Source: CAD feature listing. Evaluate the final solid. Frame: model axes, mm. Round coordinates to 2 decimals unless told otherwise and drop trailing zeros. Write each loop counter-clockwise with the first axis right and the second up, starting at its lowest first coordinate (ties: lowest second). Pieces come first, ordered by that corner, then holes. Notation, with made-up numbers: M 8,65 L 66,65 A31 cw 66,89 Z; hole C -1.5,13.5 d6. An arc over 180 degrees is marked long. Answer in a Markdown table with one row per item.
from build123d import *

# Parameters (mm, degrees)
SKETCH_1_R               = 32
SKETCH_1_R_2             = 5
EXTRUDE_1_DEPTH          = 4
SKETCH_2_R               = 2.05
CUT_EXTRUDE_1_DEPTH      = 5
SKETCH_3_R               = 24
CUT_EXTRUDE_2_DEPTH      = 10
PATTERN_CIRCULAR_1_COUNT = 6
SKETCH_4_R               = 1.6
CUT_EXTRUDE_3_DEPTH      = 23
PATTERN_CIRCULAR_2_COUNT = 6
FILLET_1_R               = 3


# Read off the part's stored shape, not the designer's step: 高级异型孔2
with BuildPart() as part:
    # 草图1 → 凸台-拉伸1 (new body)
    with BuildSketch(Plane.XY):
        Circle(SKETCH_1_R)
        Circle(SKETCH_1_R_2, mode=Mode.SUBTRACT)
    extrude(amount=EXTRUDE_1_DEPTH)

    # 草图2 → 切除-拉伸1 (cut)
    with BuildSketch(Plane.XY.offset(4)):
        with Locations((0, 12)):
            Circle(SKETCH_2_R)
        with Locations((0, -12)):
            Circle(SKETCH_2_R)
    extrude(amount=-CUT_EXTRUDE_1_DEPTH, mode=Mode.SUBTRACT)

    # 草图3 → 切除-拉伸2 (cut)
    with BuildSketch(Plane.XY.offset(4)):
        with Locations((0, 50)):
            Circle(SKETCH_3_R)
    cut_extrude_2 = extrude(amount=-CUT_EXTRUDE_2_DEPTH, mode=Mode.SUBTRACT)

    # 阵列(圆周)1: 切除-拉伸2 ×6 about axis
    pattern_circular_1_axis = Axis((0, 0, 0), (0, 0, 1))
    for i in range(1, PATTERN_CIRCULAR_1_COUNT):
        add(cut_extrude_2.rotate(pattern_circular_1_axis, i * 360 / PATTERN_CIRCULAR_1_COUNT), mode=Mode.SUBTRACT)

    # 草图4 → 切除-拉伸3 (cut)
    with BuildSketch(Plane.XY.offset(4)):
        with Locations((13.75, 23.815698604)):
            Circle(SKETCH_4_R)
    cut_extrude_3 = extrude(amount=-CUT_EXTRUDE_3_DEPTH, mode=Mode.SUBTRACT)

    # 阵列(圆周)2: 切除-拉伸3 ×6 about axis
    pattern_circular_2_axis = Axis((0, 0, 0), (0, 0, 1))
    for i in range(1, PATTERN_CIRCULAR_2_COUNT):
        add(cut_extrude_3.rotate(pattern_circular_2_axis, i * 360 / PATTERN_CIRCULAR_2_COUNT), mode=Mode.SUBTRACT)

    # 圆角1
    fillet_1_edges = [part.edges().sort_by_distance(p)[0] for p in [
        (-12.447071945, 29.48, 2),
        (12.447071945, 29.48, 2),
        (-31.753964876, 3.960519493, 2),
        (-19.306892931, 25.519480507, 2),
        (19.306892931, 25.519480507, 2),
        (31.753964876, 3.960519493, 2),
        (31.753964876, -3.960519493, 2),
        (19.306892931, -25.519480507, 2),
        (-19.306892931, -25.519480507, 2),
        (-31.753964876, -3.960519493, 2),
        (12.447071945, -29.48, 2),
        (-12.447071945, -29.48, 2),
    ]]
    fillet(fillet_1_edges, radius=FILLET_1_R)

    # 高级异型孔2 outline → 高级异型孔2 (revolve, cut)
    with BuildSketch(Plane.XZ.offset(12)):
        Polygon((2.25, 2.05), (2.05, 2.05), (2.05, 0), (4.3, 0), align=None)
    revolve(axis=Axis((0, -12, 0), (0, 0, 1)), mode=Mode.SUBTRACT)

    # Other 2 2 outline → Other 2 2 (revolve, cut)
    with BuildSketch(Plane.XZ.offset(-12)):
        Polygon((2.25, 2.05), (2.05, 2.05), (2.05, 0), (4.3, 0), align=None)
    revolve(axis=Axis((0, 12, 0), (0, 0, 1)), mode=Mode.SUBTRACT)


solid = part.part
Q1. Pull-direction query (Y, two-part tool) for faces 1 (the cylindrical face through (22.436, 13.142, 2.028)), 2 (the cylindrical face through (-16.029, -27.696, 1.972)), 3 (the cylindrical face through (-26.02, -0.61, 2.03)); classes: pulls with the +Y half, pulls with the -Y half, needs draft (parallel to the pull), parting line crosses it, or undercut.
Solutions:
| item | result |
|---|---|
| face 1 | pulls with the +Y half |
| face 2 | pulls with the -Y half |
| face 3 | undercut |
Q2. Section C-C (z = 2.75). State how many separate pieces and enclosed holes the cut face has, and give its area (3 significant figures).
Solutions:
| item | result |
|---|---|
| separate pieces | 1 |
| enclosed holes | 9 |
| area | 2,450 mm2 |
Q3. Contact query for flat-ended pins moving along their axis: pin 1 Ø3.5 at (x, y) = (-27.5, 0) entering from -Z; pin 2 Ø1 at (x, z) = (-10, 0.5) entering from +Y; pin 3 Ø2 at (x, z) = (19, 1) entering from -Y. Output: stop coordinate, or through.
Solutions:
| item | result |
|---|---|
| pin 1 | stops at z = 0 |
| pin 2 | stops at y = 28.42 |
| pin 3 | stops at y = -26.46 |
Q4. Section B-B (x = -27.5). Return loops of the section in (y, z), and give its area (3 significant figures).
Solutions:
| item | result |
|---|---|
| outline | M -6.94,0 L -1.6,0 L -1.6,4 L -6.94,4 Z; M 1.6,0 L 6.94,0 L 6.94,4 L 1.6,4 Z |
| area | 42.7 mm2 |
Q5. Section A-A (y = -12). Return loops of the section in (x, z), and give its area (3 significant figures).
Solutions:
| item | result |
|---|---|
| outline | M -23.13,0 L -4.3,0 L -2.25,2.05 L -2.05,2.05 L -2.05,4 L -23.13,4 Z; M 2.05,2.05 L 2.25,2.05 L 4.3,0 L 23.13,0 L 23.13,4 L 2.05,4 Z |
| area | 164 mm2 |
Q6. Material intervals for probe 1 along Y at (x, z) = (0, 2.85); probe 2 along Y at (x, z) = (-13.75, 2.4); probe 3 along Y at (x, z) = (-27.5, 1.95), sorted ascending.
Solutions:
| item | result |
|---|---|
| probe 1 | y = -26 to -14.05, -9.95 to -5, 5 to 9.95, 14.05 to 26 |
| probe 2 | y = -28.89 to -25.42, -22.22 to 22.22, 25.42 to 28.89 |
| probe 3 | y = -6.94 to -1.6, 1.6 to 6.94 |
